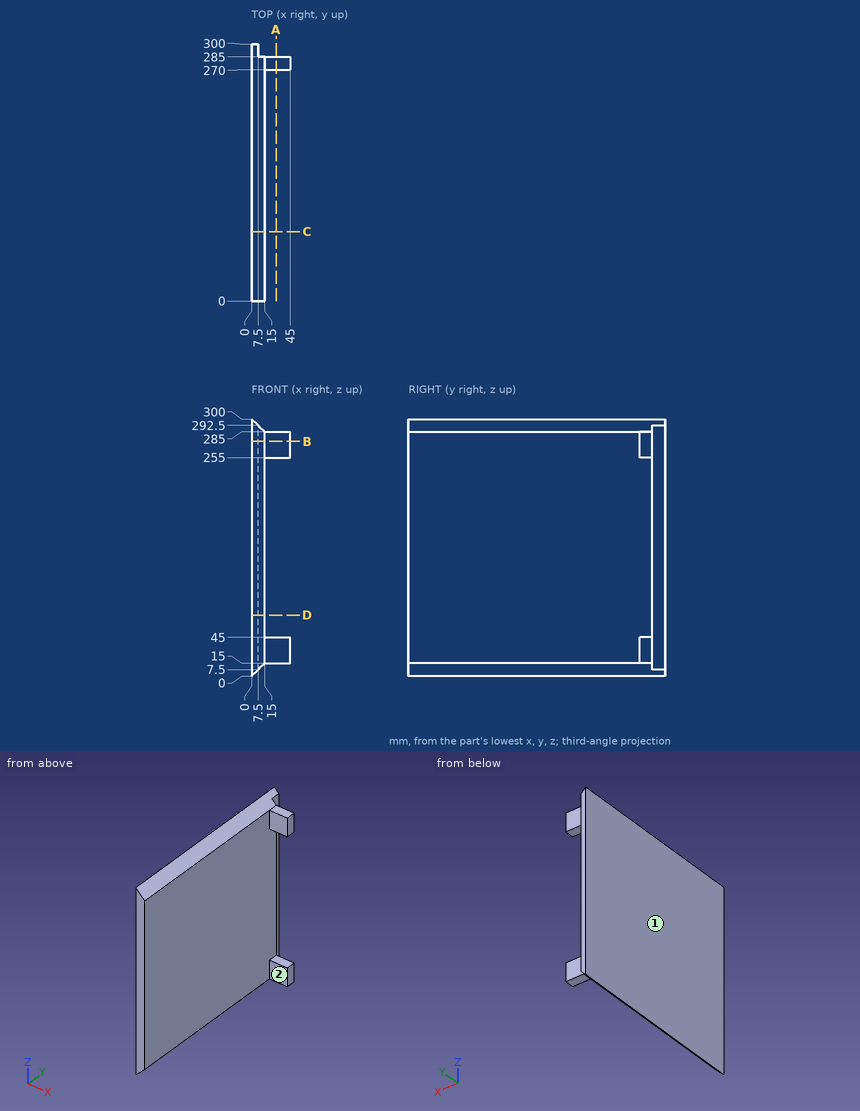
Job drawing, mm, ordinate dimensions from the low corner. One solid piece. Give positions to 0.01 mm unless a question says otherwise; leave off trailing zeros. Write each loop counter-clockwise with the first axis right and the second up, starting at its lowest first coordinate (ties: lowest second). Pieces come first, ordered by that corner, then holes. Notation, with made-up numbers: M 13,4 L 34,4 A22 ccw 34,37 Z; hole C 80,20 d8. An arc over 180 degrees is marked long. One line per item, written item: value. Start each with the question number.
Q1. Two-plate mould, pull along Y, no slides. Class the marked faces 1 and 2: +Y half, -Y half, draft (parallel to the pull), parting line (faces both ways), or undercut.
Q2. Saw through at C-C, the plane y = 81. Write the cut outline in (x, z).
Q3. Probe probe 1 along X at (y, z) = (186, 19.5); probe 2 along Y at (x, z) = (8.5, 173.5); probe 3 along Y at (x, z) = (31.5, 36.5). List the from-to ranges inside material, lowest first. Write a range as [from, to].
Q4. Saw through at B-B, the plane z = 274. Write the cut outline in (x, y), plus the area to 3 significant figures.
Q5. Saw through at D-D, the plane z = 71. Write the cut outline in (x, y), plus the area to 3 significant figures.
Q6. Saw through at A-A, the plane x = 28.5. Write the cut outline in (y, z), plus the area to 3 significant figures.
Q7. Drop flat-ended pins along their axis: pin 1 Ø6 at (x, z) = (32.5, 38) entering from -Y; pin 2 Ø16.5 at (x, y) = (32.5, 279) entering from +Z; pin 3 Ø7.5 at (x, y) = (32, 280.5) entering from -Z. Give the stop position or say it passes through.
Output values:
1. face 1: draft
1. face 2: -Y half
2. outline: M 0,0 L 15,15 L 15,285 L 0,300 Z
3. probe 1: x = [0, 15]
3. probe 2: y = [0, 285]
3. probe 3: y = [270, 285]
4. outline: M 0,0 L 15,0 L 15,270 L 45,270 L 45,285 L 7.5,285 L 7.5,300 L 0,300 Z
4. area: 4,840 mm²
5. outline: M 0,0 L 15,0 L 15,285 L 7.5,285 L 7.5,300 L 0,300 Z
5. area: 4,390 mm²
6. outline: M 270,15 L 285,15 L 285,45 L 270,45 Z; M 270,255 L 285,255 L 285,285 L 270,285 Z
6. area: 900 mm²
7. pin 1: stops at y = 270
7. pin 2: stops at z = 285
7. pin 3: stops at z = 15
